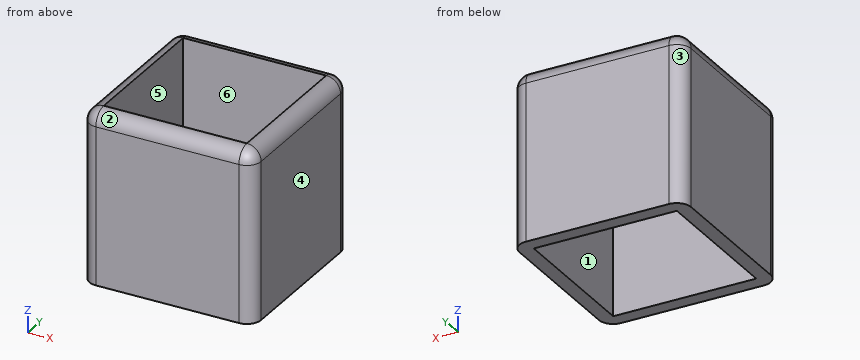
from build123d import *

# Parameters (mm, degrees)
F0_W        = 60
F0_H        = 60
F1_DEPTH    = 60
F2_R        = 5
F3_T1_DEPTH = 67.5
F3_S5_W     = 5
F3_S5_H     = 5
F3_T6_DEPTH = 5
F4_T        = 5
F5_DEPTH    = 12.5


# Not quite as in the source:
# - a fillet or chamfer that OpenCascade refuses, or shapes differently, is made with other operations: its cross-section is extruded or revolved along the edge and cut away or added
# - a shell that OpenCascade refuses in one call is made with other operations: the cavity is built on its own and cut out


with BuildPart() as f1:
    # F0 (on Top) → F1 (new body)
    with BuildSketch(Plane.XY):
        with Locations((17.446616729, -1.6685388982)):
            Rectangle(F0_W, F0_H)
    extrude(amount=F1_DEPTH)

    # F2
    f2_edges = [f1.edges().sort_by_distance(p)[0] for p in [
        (17.446617, -31.668539, 60),
        (47.446617, -1.668539, 60),
        (-12.553383, -1.668539, 60),
        (17.446617, 28.331461, 60),
        (47.446617, 28.331461, 30),
        (47.446617, -31.668539, 30),
        (-12.553383, 28.331461, 30),
    ]]
    fillet(f2_edges, radius=F2_R)

    # F3: fillet of radius 5 on 1 edges, made by hand

    # F3_s2 → F3_t1 (cut)
    with BuildSketch(Plane.XY.offset(-12.5)):
        with BuildLine():
            ThreePointArc((-12.553383271, -26.6685388982), (-11.0889171769, -30.2040728042), (-7.553383271, -31.6685388982))
            Line((-7.553383271, -31.6685388982), (-12.553383271, -31.6685388982))
            Line((-12.553383271, -31.6685388982), (-12.553383271, -26.6685388982))
        make_face()
    extrude(amount=F3_T1_DEPTH, mode=Mode.SUBTRACT)


with BuildPart() as f3_tool4:
    # F3_s5 → F3_t6 (new body)
    with BuildSketch(Plane.YZ.offset(-7.553383271)):
        with Locations((-29.1685388982, 57.5)):
            Rectangle(F3_S5_W, F3_S5_H)
    extrude(amount=-F3_T6_DEPTH)

    # F3_s7 → F3_t8 (revolve, cut)
    with BuildSketch(Plane(origin=(-7.553383271, -26.6685388982, 55), x_dir=(0, 0.7071067812, -0.7071067812), z_dir=(0, 0.7071067812, 0.7071067812))):
        with BuildLine():
            ThreePointArc((0, -5), (5, 0), (0, 5))
            Line((0, 5), (0, -5))
        make_face()
    revolve(axis=Axis((-7.553383271, -26.6685388982, 55), (-1, 0, 0)), mode=Mode.SUBTRACT)


with BuildPart() as f1_1:
    add(f1.part)

    # F3_t3: cut F3_tool4
    add(f3_tool4.part, mode=Mode.SUBTRACT)

    # F4: shell of thickness 5, made by hand


with BuildPart() as f4_core1:
    # F4_t2: copy of F1
    add(f1_1.part)

    # the walls: a layer under each face that stays
    f4_faces = [f4_core1.faces().sort_by_distance(p)[0] for p in [
        (17.446616729, 28.3314611018, 27.5),
        (47.446616729, -1.6685388982, 27.5),
        (17.446616729, -31.6685388982, 27.5),
        (-12.553383271, -1.6685388982, 27.5),
        (17.446616729, -1.6685388982, 60),
    ]]
    thicken(f4_faces, amount=-F4_T, mode=Mode.SUBTRACT)


with BuildPart() as f1_2:
    add(f1_1.part)

    # what is left inside the walls is the cavity
    f4_cavity = [f4_core1.part.solids().sort_by_distance(p)[0] for p in [
        (42.396617, -1.668539, 36.666667),
    ]]
    add(f4_cavity, mode=Mode.SUBTRACT)

    # F5 (cut, symmetric): a face of the model
    f5_faces = [f1_2.faces().sort_by_distance(p)[0] for p in [
        (17.446616729, -1.6685388982, 60),
    ]]
    extrude(f5_faces, amount=F5_DEPTH, both=True, mode=Mode.SUBTRACT)


solid = f1_2.part
The listing builds one solid part. Answer for the finished solid, in the listing's coordinates (mm). Face numbers are marked on the shaded views. A direction names the side the tool comes from. Round coordinates to 2 decimals unless told otherwise and drop trailing zeros. Write each loop counter-clockwise with the first axis right and the second up, starting at its lowest first coordinate (ties: lowest second). Pieces come first, ordered by that corner, then holes. Notation, with made-up numbers: M 36,-34.5 L 40,-34.5 A20 cw 40,-20.5 Z; hole C 16,79 d7. An arc over 180 degrees is marked long. Write each question's results on one line, items separated by ' | '. Start each with the question number.
Item 1: For a pull along Y with two mould halves and no side action, classify the marked faces 3, 4, 5 and 6 as pulls with the +Y half, pulls with the -Y half, needs draft (parallel to the pull), parting line crosses it, or undercut.
Item 2: A cutting plane is placed at B-B on z = 5. Write down the section's boundary in (x, y), and give its area (3 significant figures).
Item 3: A cutting plane is placed at C-C on y = 15. Write down the section's boundary in (x, z).
Item 4: For the marked faces 1 and 2, determine the directions among +Z, -Z, +X, -X, +Y, -Y from which every point of the face is accessible in a straight line to the end or side of a thin tool.
Item 5: A cutting plane is placed at A-A on x = 36. Write down the section's boundary in (y, z), and give its area (3 significant figures).
Item 6: Straight lines are drawn through the part: L1, parallel to X at y = 11.5, z = 16; L2, parallel to Y at x = 27, z = 45.5; L3, parallel to Y at x = 40, z = 56.5. For each, find the intervals that lie inside material, in ascending order. Write a range as [from, to].
Check sheet entries:
1) face 3: pulls with the +Y half | face 4: needs draft | face 5: undercut | face 6: undercut
2) outline: M -12.55,-26.67 A5 ccw -7.55,-31.67 L 42.45,-31.67 A5 ccw 47.45,-26.67 L 47.45,23.33 A5 ccw 42.45,28.33 L -7.55,28.33 A5 ccw -12.55,23.33 Z; hole M -7.55,-26.67 L 42.45,-26.67 L 42.45,23.33 L -7.55,23.33 Z | area: 1,080 mm²
3) outline: M -12.55,0 L -7.55,0 L -7.55,60 A5 ccw -12.55,55 Z; M 42.45,0 L 47.45,0 L 47.45,55 A5 ccw 42.45,60 Z
4) face 1: +Z, -Z | face 2: +Z, +X, -X, -Y
5) outline: M -31.67,0 L -26.67,0 L -26.67,60 A5 ccw -31.67,55 Z; M 23.33,0 L 28.33,0 L 28.33,55 A5 ccw 23.33,60 Z | area: 589 mm²
6) L1: [-12.55, -7.55], [42.45, 47.45] | L2: [-31.67, -26.67], [23.33, 28.33] | L3: [-31.44, -26.67], [23.33, 28.1]
